Design review of the part built by this model. Coordinates are the model's own, in mm. A direction names the side the tool comes from. Round coordinates to 2 decimals unless told otherwise and drop trailing zeros. Write each loop counter-clockwise with the first axis right and the second up, starting at its lowest first coordinate (ties: lowest second). Pieces come first, ordered by that corner, then holes.
from build123d import *

# Parameters (mm, degrees)
F1_DEPTH = 22.225
F2_R     = 3.740582
F3_R     = 3.5687
F4_DEPTH = 4.8006


with BuildPart() as f1:
    # F0 (on Front) → F1 (new body)
    with BuildSketch(Plane.XZ):
        Polygon((4.8006, 34.427944), (0, 34.427944), (0, -16.448256), (25.3238, -16.448256), (25.3238, -11.647656), (4.8006, -11.647656), align=None)
    extrude(amount=F1_DEPTH)

    # F2
    f2_edges = [f1.edges().sort_by_distance(p)[0] for p in [
        (4.8006, -11.1125, 34.427944),
        (4.8006, -11.1125, -11.647656),
        (25.3238, -11.1125, -11.647656),
    ]]
    fillet(f2_edges, radius=F2_R)

    # F3 (on face) → F4 (cut)
    with BuildSketch(Plane(origin=(0, 0, 0), x_dir=(0, -1, 0), z_dir=(-1, 0, 0))):
        with Locations((11.1125, 21.689844)):
            Circle(F3_R)
        with Locations((11.1125, -3.735556)):
            Circle(F3_R)
    extrude(amount=-F4_DEPTH, mode=Mode.SUBTRACT)


solid = f1.part
1) For P1, Ø2, axis at y = -20, z = 7, coming from the +X side; P2, Ø5, axis at x = 8.5, z = 27, coming from the -Y side; P3, Ø1, axis at x = 19, y = -12.5, coming from the +Z side, all flat-tipped, find the tip position at first contact; note any pin that passes through.
2) For line 1 along Z through (x, y) = (3.5, -11.25); line 2 along X through (y, z) = (-16.5, 7.5); line 3 along Z through (x, y) = (19.75, -7.5), list the stretches that pass through material, from the lowest coordinate up.
3) The part is to be moulded in two halves that separate along Y. For faces 1 (the face through (4, -22.225, 3)), 2 (the face through (2.367, -8.281, -5.907)), 3 (the face through (4, 0, 3)), say which applies: pulls with the +Y half, pulls with the -Y half, needs draft (parallel to the pull), parting line crosses it, or undercut.
4) Add section C-C on y = -10.75. State the section outline as (x, z) points, and give its area (3 significant figures).
5) Add section A-A on y = -18.75. State the section outline as (x, z) points, and give its area (3 significant figures).
6) Add section B-B on z = 20. State the section outline as (x, y) points (3 decimals).
7) For faces 4 (the face through (25.324, -11, -16)), 5 (the face through (15, -11, -11.648)), list the 3-axis set-ups (+Z, -Z, +X, -X, +Y, -Y) from which the entire face can be reached by the end or side of a thin tool; tool diameter is ignored.
8) Add section D-D on x = 14.25. State the section outline as (y, z) points (3 decimals).
Computed:
1. P1: stops at x = 4.8
1. P2: passes through
1. P3: stops at z = -11.65
2. line 1: z = -16.45 to -7.3, -0.17 to 18.12, 25.26 to 33.52
2. line 2: x = 0 to 4.8
2. line 3: z = -16.45 to -11.65
3. face 1: pulls with the -Y half
3. face 2: undercut
3. face 3: pulls with the +Y half
4. outline: (0, -16.45) - (25.32, -16.45) - (25.32, -15.39) arc R3.74 ccw to (21.58, -11.65) - (8.54, -11.65) arc R3.74 cw to (4.8, -7.91) - (4.8, -7.29) - (0, -7.29) - close; (0, -0.19) - (4.8, -0.19) - (4.8, 18.14) - (0, 18.14) - close; (0, 25.24) - (4.8, 25.24) - (4.8, 30.69) arc R3.74 ccw to (1.06, 34.43) - (0, 34.43) - close
4. area: 272 mm2
5. outline: (0, -16.45) - (25.32, -16.45) - (25.32, -15.39) arc R3.74 ccw to (21.58, -11.65) - (8.54, -11.65) arc R3.74 cw to (4.8, -7.91) - (4.8, 30.69) arc R3.74 ccw to (1.06, 34.43) - (0, 34.43) - close
5. area: 340 mm2
6. outline: (0, -22.225) - (4.801, -22.225) - (4.801, -14.256) - (0, -14.256) - close; (0, -7.969) - (4.801, -7.969) - (4.801, 0) - (0, 0) - close
7. face 4: +Z, -Z, +X, +Y, -Y
7. face 5: +Z, +X, +Y, -Y
8. outline: (-22.225, -16.448) - (0, -16.448) - (0, -11.648) - (-22.225, -11.648) - close
